Part model, mm, in its own coordinate system. A direction names the side the tool comes from. Round coordinates to 2 decimals unless told otherwise and drop trailing zeros. Loops run counter-clockwise (first coordinate to the right, second up) from the corner with the lowest first, then second, coordinate; pieces in that order, holes last.
(1) Flat gauge pins, fed straight in: pin 1 (25 mm diameter, centred on x = 12, y = 3, fed in from +Z); pin 2 (3.5 mm diameter, centred on x = 3.37, z = 0, fed in from -Y); pin 3 (1.9 mm diameter, centred on x = -3.37, z = 0, fed in from -Y); pin 4 (15 mm diameter, centred on x = -10.5, y = 9.5, fed in from -Z). Where does each tip first touch, or does it go through?
(2) Cut at B-B on x = 3. Count the separate pieces of the cut face and the enclosed holes in it, then the cut area to 3 significant figures.
(3) Cut at A-A on y = 0. List the corners of the cut face in (x, z), then the cut area to 3 significant figures.
(4) Tool access for faces 1 (the face through (-3.604, 26.263, -1.045)), 2 (the face through (0.93, -22.88, -0.01)), 3 (the face through (8.7, -21.4, 1)): list every direction of +Z, -Z, +X, -X, +Y, -Y with a clear straight run to the whole face (end or side of a thin tool).
(5) Probe probe 1 along Y at (x, z) = (8.5, -0.75); probe 2 along Y at (x, z) = (15.5, 2); probe 3 along X at (y, z) = (3.5, -2.25). List the from-to ranges inside material, lowest first.
(6) Mould opens along Z. For faces 4 (the face through (17, -19, 3.839)), 5 (the face through (0, -25, 0)), 6 (the face through (-17, -19, -3.839)) say: +Z half, -Z half, draft (parallel to the pull), parting line (faces both ways), or undercut.
from build123d import *

# Parameters (mm, degrees)
F5_R           = 2
F1_R           = 1.0708620531
F6_DEPTH       = 43.9
F7_ANGLE_START = 100
F7_ANGLE       = 157
F8_ANGLE_BACK  = 77
F8_ANGLE       = 177
F9_DEPTH       = 25


with BuildPart() as f2:
    # F1 (on Front) → F2 (revolve)
    with BuildSketch(Plane.XZ):
        with BuildLine():
            ThreePointArc((-25.1082326719, -3.8388347315), (-25.4, 0), (-25.1082326719, 3.8388347315))
            Line((-25.1082326719, 3.8388347315), (-27.6482326719, 3.8388347315))
            Line((-27.6482326719, 3.8388347315), (-27.6482326719, -3.8388347315))
            Line((-27.6482326719, -3.8388347315), (-25.1082326719, -3.8388347315))
        make_face()
    revolve(axis=Axis((0, 0, 0.0089984387), (0, 0, -1)))

    # F5
    f5_edges = [f2.edges().sort_by_distance(p)[0] for p in [
        (27.648233, 0, 3.838835),
        (27.648233, 0, -3.838835),
    ]]
    fillet(f5_edges, radius=F5_R)

    # F1 (on Front) → F6 (cut)
    with BuildSketch(Plane.XZ):
        with Locations((3.3717958722, 0)):
            Circle(F1_R)
        with Locations((-3.3717958722, 0)):
            Circle(F1_R)
    extrude(amount=-F6_DEPTH, mode=Mode.SUBTRACT)

    # F1 (on Front) → F7 (revolve)
    with BuildSketch(Plane.XZ, mode=Mode.PRIVATE) as f7_sk:
        with BuildLine():
            ThreePointArc((25.3803073267, -1), (25.3950763545, -0.5000969409), (25.4, 0))
            ThreePointArc((25.4, 0), (25.3950763545, 0.5000969409), (25.3803073267, 1))
            Line((25.3803073267, 1), (22.9, 1))
            Line((22.9, 1), (22.9, -1))
            Line((22.9, -1), (25.3803073267, -1))
        make_face()
    revolve(f7_sk.sketch.rotate(Axis((0, 0, 0.0089984387), (0, 0, -1)), F7_ANGLE_START), axis=Axis((0, 0, 0.0089984387), (0, 0, -1)), revolution_arc=F7_ANGLE)

    # F1 (on Front) → F8 (revolve)
    with BuildSketch(Plane.XZ, mode=Mode.PRIVATE) as f8_sk:
        with BuildLine():
            ThreePointArc((25.3803073267, -1), (25.3950763545, -0.5000969409), (25.4, 0))
            ThreePointArc((25.4, 0), (25.3950763545, 0.5000969409), (25.3803073267, 1))
            Line((25.3803073267, 1), (22.9, 1))
            Line((22.9, 1), (22.9, -1))
            Line((22.9, -1), (25.3803073267, -1))
        make_face()
    revolve(f8_sk.sketch.rotate(Axis((0, 0, 0.0089984387), (0, 0, -1)), -F8_ANGLE_BACK), axis=Axis((0, 0, 0.0089984387), (0, 0, -1)), revolution_arc=F8_ANGLE)

    # F1 (on Front) → F9 (cut)
    with BuildSketch(Plane.XZ):
        with BuildLine():
            Line((0, -0.700821599), (0, 0.700821599))
            ThreePointArc((0, 0.700821599), (-0.700821599, 0), (0, -0.700821599))
        make_face()
        with BuildLine():
            ThreePointArc((0.700821599, 0), (0.4955557051, 0.4955557051), (0, 0.700821599))
            Line((0, 0.700821599), (0, -0.700821599))
            ThreePointArc((0, -0.700821599), (0.4955557051, -0.4955557051), (0.700821599, 0))
        make_face()
    extrude(amount=F9_DEPTH, mode=Mode.SUBTRACT)


solid = f2.part
Final values:
1. pin 1: stops at z = 1
1. pin 2: stops at y = -27.6
1. pin 3: stops at y = -27.54
1. pin 4: passes through
2. separate pieces: 3
2. enclosed holes: 0
2. area: 33.3 mm2
3. outline: (-27.65, -1.84) arc R2 ccw to (-25.65, -3.84) - (-25.11, -3.84) arc R25.4 cw to (-25.38, -1) - (-22.9, -1) - (-22.9, 1) - (-25.38, 1) arc R25.4 cw to (-25.11, 3.84) - (-25.65, 3.84) arc R2 ccw to (-27.65, 1.84) - close; (22.9, -1) - (25.38, -1) arc R25.4 cw to (25.11, -3.84) - (25.65, -3.84) arc R2 ccw to (27.65, -1.84) - (27.65, 1.84) arc R2 ccw to (25.65, 3.84) - (25.11, 3.84) arc R25.4 cw to (25.38, 1) - (22.9, 1) - close
3. area: 42.6 mm2
4. face 1: +Y
4. face 2: +Z, -Z
4. face 3: none
5. probe 1: y = -26.31 to -21.26, 21.26 to 26.31
5. probe 2: y = -22.89 to -20.02, 20.02 to 22.89
5. probe 3: x = -27.38 to -25.06, 25.06 to 27.38
6. face 4: +Z half
6. face 5: undercut
6. face 6: -Z half
